CAD build for the part. Positions are in the model's coordinates, mm. Round coordinates to 2 decimals unless told otherwise and drop trailing zeros. Loops run counter-clockwise (first coordinate to the right, second up) from the corner with the lowest first, then second, coordinate; pieces in that order, holes last. Notation, with made-up numbers: (55, 23.25) - (80, 23.25) arc R9 cw to (80, 35.25) - close; hole circle Ø6 at (5, 4.25). An arc over 180 degrees is marked (long way). Use one line per item in the form item = value.
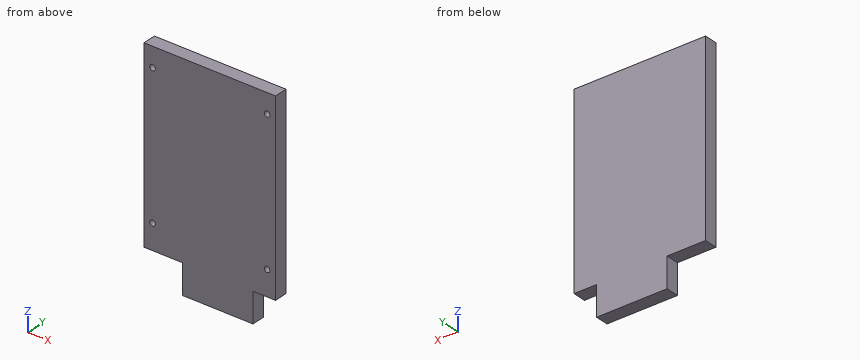
from build123d import *

# Parameters (mm, degrees)
SKETCH1_W           = 70
SKETCH1_H           = 100
BOSS_EXTRUDE1_DEPTH = 7
SKETCH2_R           = 1.5
CUT_EXTRUDE1_DEPTH  = 5
SKETCH3_W           = 37.5
SKETCH3_H           = 16
BOSS_EXTRUDE2_DEPTH = 7


with BuildPart() as part:
    # Sketch1 → Boss-Extrude1 (new body)
    with BuildSketch(Plane(origin=(0, 0, 0), x_dir=(1, 0, 0), z_dir=(0, 1, 0))):
        Rectangle(SKETCH1_W, SKETCH1_H)
    extrude(amount=BOSS_EXTRUDE1_DEPTH)

    # Sketch2 → Cut-Extrude1 (cut)
    with BuildSketch(Plane.XZ):
        with Locations(Location((-30.5, -36.5, 0), (0, 0, 270))):
            Circle(SKETCH2_R)
        with Locations(Location((-30.5, 39.5, 0), (0, 0, 270))):
            Circle(SKETCH2_R)
        with Locations(Location((30.5, 39.5, 0), (0, 0, 270))):
            Circle(SKETCH2_R)
        with Locations(Location((30.5, -36.5, 0), (0, 0, 270))):
            Circle(SKETCH2_R)
    extrude(amount=-CUT_EXTRUDE1_DEPTH, mode=Mode.SUBTRACT)

    # Sketch3 → Boss-Extrude2 (add)
    with BuildSketch(Plane.XZ):
        with Locations((4.25, -58)):
            Rectangle(SKETCH3_W, SKETCH3_H)
    extrude(amount=-BOSS_EXTRUDE2_DEPTH)


solid = part.part
1) Drill centre lines: probe 1 along X at (y, z) = (2.2, -36.5); probe 2 along X at (y, z) = (6, -52); probe 3 along Z at (x, y) = (-18, 3). Where is each one in solid material? Low to high.
Report:
probe_1 = -35 to -32, -29 to 29, 32 to 35
probe_2 = -14.5 to 23
probe_3 = -50 to 50
2) Slice it at B-B (z = 39.5). Write the cut outline in (x, y), plus the area to 3 significant figures.
Report:
outline = (-35, 0) - (-32, 0) - (-32, 5) - (-29, 5) - (-29, 0) - (29, 0) - (29, 5) - (32, 5) - (32, 0) - (35, 0) - (35, 7) - (-35, 7) - close
area = 460 mm^2
3) Flat gauge pin, fed straight in: pin 1 (0.9 mm diameter, centred on x = 30.5, z = -36, fed in from -Y). Where does the tip first touch, or does it go through?
Report:
pin_1 = 5
4) Slice it at A-A (x = 30.5). Write the cut outline in (y, z), plus the area to 3 significant figures.
Report:
outline = (0, -50) - (7, -50) - (7, 50) - (0, 50) - (0, 41) - (5, 41) - (5, 38) - (0, 38) - (0, -35) - (5, -35) - (5, -38) - (0, -38) - close
area = 670 mm^2
5) Slice it at C-C (x = -19). Write the cut outline in (y, z), plus the area to 3 significant figures.
Report:
outline = (0, -50) - (7, -50) - (7, 50) - (0, 50) - close
area = 700 mm^2
